Input: part model. Units: mm. Frame: model coordinates. A direction names the side the tool comes from. Give positions to 0.01 mm unless a question says otherwise; leave off trailing zeros. Order: outer loops, then holes, each group sorted by start corner. A loop starts at its lowest first (then second) coordinate and runs counter-clockwise, first axis right, second up. Notation, with made-up numbers: M 68,4 L 103,4 A15 cw 103,14 Z; hole C -24.5,82 d2. An arc over 180 degrees is marked long. Use a Markdown table: item, result.
from build123d import *

# Parameters (mm, degrees)
SKETCH1_W           = 43
SKETCH1_H           = 45.5
SKETCH1_R           = 1.75
BOSS_EXTRUDE1_DEPTH = 1
SKETCH2_W           = 40
SKETCH2_H           = 34
BOSS_EXTRUDE2_DEPTH = 3.5
CUT_EXTRUDE1_DEPTH  = 0.3


with BuildPart() as part:
    # Sketch1 → Boss-Extrude1 (new body)
    with BuildSketch(Plane.XY):
        Rectangle(SKETCH1_W, SKETCH1_H)
        with Locations((-17, 19.95)):
            Circle(SKETCH1_R, mode=Mode.SUBTRACT)
        with Locations((17, 19.95)):
            Circle(SKETCH1_R, mode=Mode.SUBTRACT)
        with Locations((-17, -20.75)):
            Circle(SKETCH1_R, mode=Mode.SUBTRACT)
        with Locations((17, -20.75)):
            Circle(SKETCH1_R, mode=Mode.SUBTRACT)
    extrude(amount=BOSS_EXTRUDE1_DEPTH)

    # Sketch2 → Boss-Extrude2 (add)
    with BuildSketch(Plane.XY.offset(1)):
        with Locations((0, 0.25)):
            Rectangle(SKETCH2_W, SKETCH2_H)
    extrude(amount=BOSS_EXTRUDE2_DEPTH)

    # Sketch3 → Cut-Extrude1 (cut)
    with BuildSketch(Plane.XY.offset(4.5)):
        with BuildLine():
            Line((-15.5, 10.75), (15.5, 10.75))
            ThreePointArc((15.5, 10.75), (17.621320344, 9.871320344), (18.5, 7.75))
            Line((18.5, 7.75), (18.5, -12.25))
            ThreePointArc((18.5, -12.25), (17.621320344, -14.371320344), (15.5, -15.25))
            Line((15.5, -15.25), (-15.5, -15.25))
            ThreePointArc((-15.5, -15.25), (-17.621320344, -14.371320344), (-18.5, -12.25))
            Line((-18.5, -12.25), (-18.5, 7.75))
            ThreePointArc((-18.5, 7.75), (-17.621320344, 9.871320344), (-15.5, 10.75))
        make_face()
    extrude(amount=-CUT_EXTRUDE1_DEPTH, mode=Mode.SUBTRACT)


solid = part.part
1) Cut plane C-C on y = -4. Return loops of the section in (x, z).
Response values:
| item | result |
|---|---|
| outline | M -21.5,0 L 21.5,0 L 21.5,1 L 20,1 L 20,4.5 L 18.5,4.5 L 18.5,4.2 L -18.5,4.2 L -18.5,4.5 L -20,4.5 L -20,1 L -21.5,1 Z |
2) Mould query, pull axis Y, two halves, no side actions, for faces 1 (the face through (-0.3, -22.75, 0.5)), 2 (the face through (21.5, -0.3, 0.5)), 3 (the face through (-18.4, 18.9, 0.5)). Classes: released by +Y, released by -Y, zero draft, split by the parting line, or undercut.
Response values:
| item | result |
|---|---|
| face 1 | released by -Y |
| face 2 | zero draft |
| face 3 | undercut |
3) Cut plane B-B on x = -5.5. Return loops of the section in (y, z), and give its area (3 significant figures).
Response values:
| item | result |
|---|---|
| outline | M -22.75,0 L 22.75,0 L 22.75,1 L 17.25,1 L 17.25,4.5 L 10.75,4.5 L 10.75,4.2 L -15.25,4.2 L -15.25,4.5 L -16.75,4.5 L -16.75,1 L -22.75,1 Z |
| area | 157 mm² |
4) Cut plane A-A on y = -20.75. Return loops of the section in (x, z), and give its area (3 significant figures).
Response values:
| item | result |
|---|---|
| outline | M -21.5,0 L -18.75,0 L -18.75,1 L -21.5,1 Z; M -15.25,0 L 15.25,0 L 15.25,1 L -15.25,1 Z; M 18.75,0 L 21.5,0 L 21.5,1 L 18.75,1 Z |
| area | 36.0 mm² |
5) Cut plane D-D on x = -17. Return loops of the section in (y, z).
Response values:
| item | result |
|---|---|
| outline | M -22.75,0 L -22.5,0 L -22.5,1 L -22.75,1 Z; M -19,0 L 18.2,0 L 18.2,1 L 17.25,1 L 17.25,4.5 L 10.35,4.5 L 10.35,4.2 L -14.85,4.2 L -14.85,4.5 L -16.75,4.5 L -16.75,1 L -19,1 Z; M 21.7,0 L 22.75,0 L 22.75,1 L 21.7,1 Z |
6) Material intervals for line 1 (Y direction, x = 17, z = 0.8); line 2 (Z direction, x = 8.5, y = 2); line 3 (Y direction, x = -12, z = 1.5), sorted ascending. Write a range as from..to.
Response values:
| item | result |
|---|---|
| line 1 | y = -22.75..-22.5, -19..18.2, 21.7..22.75 |
| line 2 | z = 0..4.2 |
| line 3 | y = -16.75..17.25 |
7) Reachability of faces 4 (the face through (0, -16.75, 3)), 5 (the face through (20, 0, 3)), 6 (the face through (0, -2, 4.2)), 7 (the face through (-20, 0, 3)) from +Z, -Z, +X, -X, +Y, -Y: full face, straight path, thin tool, end or side. Return the list, or none.
Response values:
| item | result |
|---|---|
| face 4 | +Z, +X, -X, -Y |
| face 5 | +Z, +X, +Y, -Y |
| face 6 | +Z |
| face 7 | +Z, -X, +Y, -Y |
8) First-contact query: pin 1 Ø1.8 at (x, z) = (2.5, 2.5) entering from +Y; pin 2 Ø2 at (y, z) = (-16, 3.5) entering from -X; pin 3 Ø1.8 at (x, z) = (-0.5, 3) entering from -Y. Flat tips, straight axial feed; report the tip coordinate or a pass-through.
Response values:
| item | result |
|---|---|
| pin 1 | stops at y = 17.25 |
| pin 2 | stops at x = -20 |
| pin 3 | stops at y = -16.75 |
